Study the drawing (mm; zero at the part's minimum x, y, z) and answer. A direction names the side the tool comes from. Coordinates: 2 decimals unless noted, no trailing zeros. Order: outer loops, then holes, each group sorted by start corner. A loop starts at its lowest first (then second) coordinate and runs counter-clockwise, first axis right, second up. Notation, with made-up numbers: M 60.5,-5.75 L 115.5,-5.75 A10 ccw 115.5,9.25 Z; hole C -3.75,38 d3. An arc over 180 degrees is marked long. Put each result on its own line as item: value.
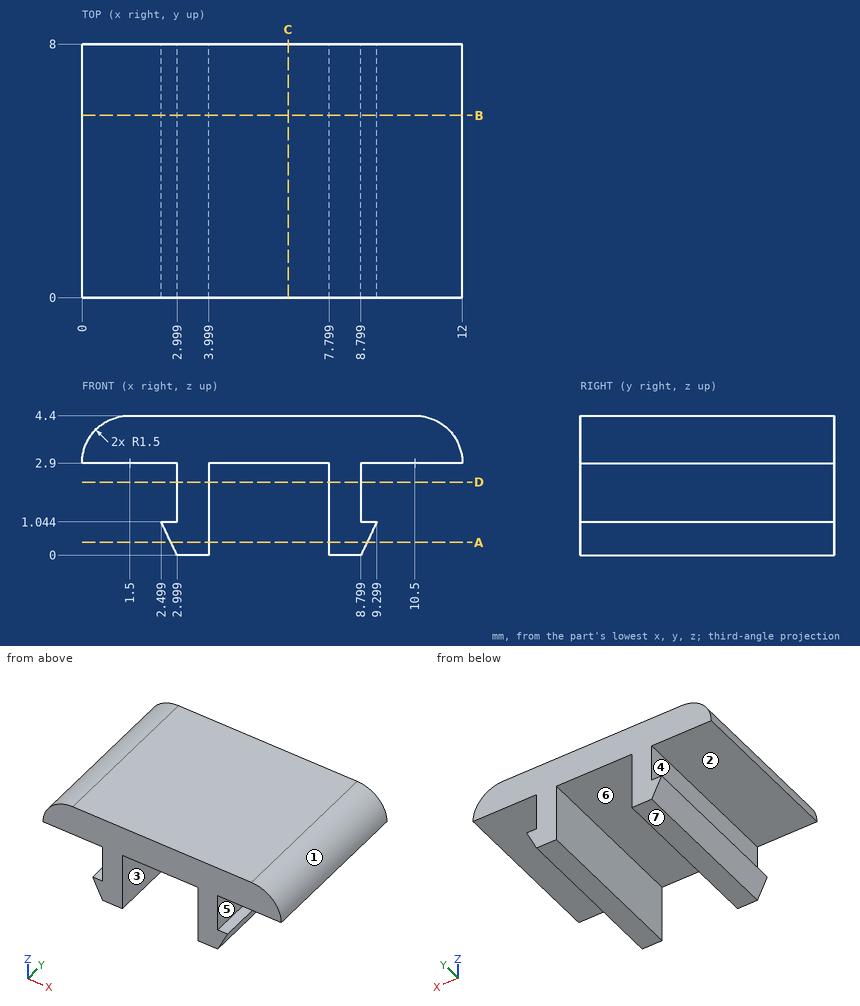
Q1. A tool of negligible diameter and unlimited length cuts with its end or side. For the marked faces 5, 6 and 7, from which of +Z, -Z, +X, -X, +Y, -Y can it reach the whole face along a straight path? Write none if from no direction.
Answers below:
face 5: +X, +Y, -Y
face 6: -Z, +Y, -Y
face 7: -Z, +X, -X, +Y, -Y
Q2. For a pull along X with two mould halves and no side action, classify the marked faces 1, 2, 3 and 4 as +X half, -X half, draft (parallel to the pull), parting line (faces both ways), or undercut.
Answers below:
face 1: +X half
face 2: draft
face 3: undercut
face 4: -X half
Q3. Find section B-B on y = 5.75. Write down the section's boundary in (x, z).
Answers below:
outline: M 0,2.9 L 3,2.9 L 3,1.04 L 2.5,1.04 L 3,0 L 4,0 L 4,2.9 L 7.8,2.9 L 7.8,0 L 8.8,0 L 9.3,1.04 L 8.8,1.04 L 8.8,2.9 L 12,2.9 A1.5 ccw 10.5,4.4 L 1.5,4.4 A1.5 ccw Z
Q4. Consider line 1 along X through (y, z) = (5.5, 1.15); line 2 along Z through (x, y) = (7.75, 7); line 3 along X through (y, z) = (0.5, 0.55) (1 decimal). Determine where each line is inside the solid, lowest interval first.
Answers below:
line 1: x = 3 to 4, 7.8 to 8.8
line 2: z = 2.9 to 4.4
line 3: x = 2.7 to 4, 7.8 to 9.1
Q5. Find section C-C on x = 6.5. Write down the section's boundary in (y, z).
Answers below:
outline: M 0,2.9 L 8,2.9 L 8,4.4 L 0,4.4 Z
Q6. Find section A-A on z = 0.4. Write down the section's boundary in (x, y).
Answers below:
outline: M 2.81,0 L 4,0 L 4,8 L 2.81,8 Z; M 7.8,0 L 8.99,0 L 8.99,8 L 7.8,8 Z
Q7. Find section D-D on z = 2.3. Write down the section's boundary in (x, y).
Answers below:
outline: M 3,0 L 4,0 L 4,8 L 3,8 Z; M 7.8,0 L 8.8,0 L 8.8,8 L 7.8,8 Z
Q8. Given pin 1 (0.9 mm diameter, centred on y = 3.5, z = 2, fed in from -X); pin 2 (1.1 mm diameter, centred on x = 6.5, y = 5.5, fed in from -Z); pin 3 (1.5 mm diameter, centred on y = 4, z = 1.5, fed in from +X); pin 4 (1.5 mm diameter, centred on x = 1.5, z = 0.5, fed in from -Y), each flat-ended and moving along its own axis, determine where each tip first touches the part or whether it passes through.
Answers below:
pin 1: stops at x = 3
pin 2: stops at z = 2.9
pin 3: stops at x = 9.3
pin 4: passes through
